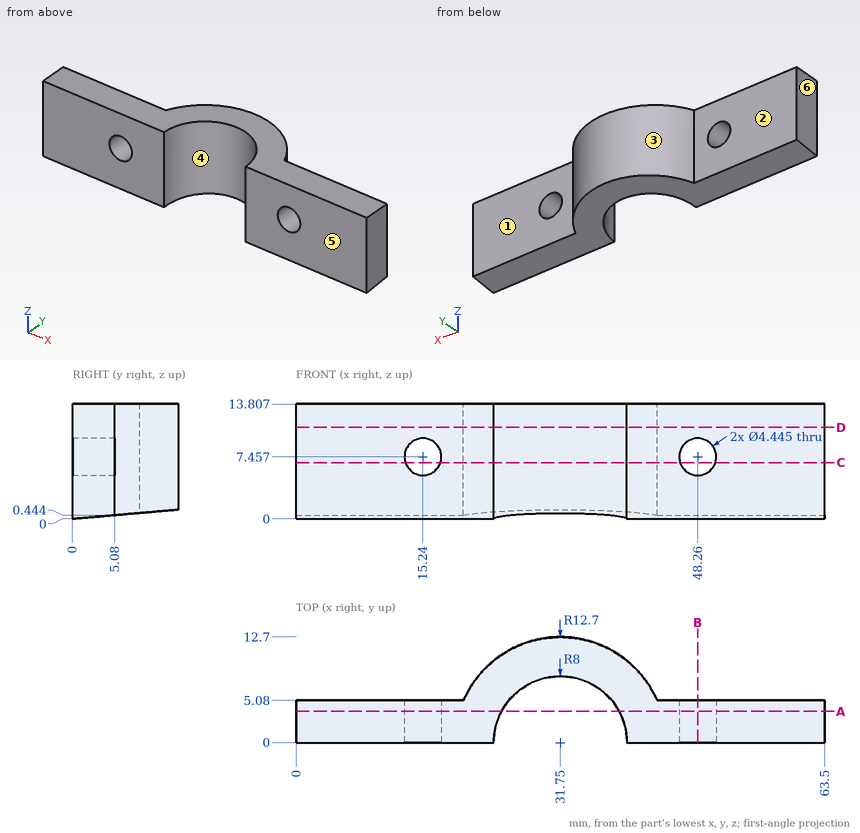
Input: dimensioned drawing with shaded views. Units: mm. Origin: part minimum x, y, z. A direction names the side the tool comes from. Coordinates: 2 decimals unless noted, no trailing zeros. Order: outer loops, then holes, each group sorted by start corner. A loop starts at its lowest first (then second) coordinate and runs counter-clockwise, first axis right, second up. Notation, with made-up numbers: M -31,49 L -2,49 A21 ccw -2,57 Z; hole C -4,82 d8. An arc over 180 degrees is marked long. Answer as CSV lines item,"result".
Q1. Section B-B on x = 48.26. Return the cut outline in (y, z) (1 decimal).
Answers:
outline,"M 0,0 L 5.1,0.4 L 5.1,5.2 L 0,5.2 Z; M 0,9.7 L 5.1,9.7 L 5.1,13.8 L 0,13.8 Z"
Q2. Draft query along X for the marked faces 4, 5 and 6. Return one class per face: pulls with the +X half, pulls with the -X half, needs draft (parallel to the pull), parting line crosses it, or undercut.
Answers:
face 4,"undercut"
face 5,"needs draft"
face 6,"pulls with the -X half"
Q3. Line query: probe 1 along X at (y, z) = (4.25, 9); probe 2 along X at (y, z) = (4.25, 5.5) (1 decimal); probe 3 along Y at (x, z) = (44, 4.25). Output: solid intervals per line, ascending. Write a range as [from, to].
Answers:
probe 1,"x = [0, 13.64], [16.84, 24.97], [38.53, 46.66], [49.86, 63.5]"
probe 2,"x = [0, 14.2], [16.3, 25], [38.5, 47.2], [49.3, 63.5]"
probe 3,"y = [0, 5.08]"
Q4. Section A-A on y = 3.75. Return the cut outline in (x, z) (1 decimal).
Answers:
outline,"M 0,0.3 L 24.7,0.3 L 24.7,13.8 L 0,13.8 Z; M 38.8,0.3 L 63.5,0.3 L 63.5,13.8 L 38.8,13.8 Z; hole C 15.2,7.5 d4.4; hole C 48.3,7.5 d4.4"
Q5. Section C-C on z = 6.75. Return the cut outline in (x, y).
Answers:
outline,"M 0,0 L 13.13,0 L 13.13,5.08 L 0,5.08 Z; M 17.35,0 L 23.75,0 A8 cw 39.75,0 L 46.15,0 L 46.15,5.08 L 43.39,5.08 A12.7 ccw 20.11,5.08 L 17.35,5.08 Z; M 50.37,0 L 63.5,0 L 63.5,5.08 L 50.37,5.08 Z"
Q6. Set-up query: the marked faces 1, 2 and 3. Return all of +Z, -Z, +X, -X, +Y, -Y with unobstructed straight access to the full face (end or side cutting, diameter ignored); none if empty.
Answers:
face 1,"+Z, -Z, +X, +Y"
face 2,"+Z, -Z, -X, +Y"
face 3,"+Z, -Z, +Y"
Q7. Section D-D on z = 11. Return the cut outline in (x, y), and give its area (3 significant figures).
Answers:
outline,"M 0,0 L 23.75,0 A8 cw 39.75,0 L 63.5,0 L 63.5,5.08 L 43.39,5.08 A12.7 ccw 20.11,5.08 L 0,5.08 Z"
area,"350 mm^2"
Q8. First-contact query: P1, Ø4, axis at y = 8.5, z = 9.5, coming from the -X side; P2, Ø6, axis at x = 35, y = 8, coming from the -Z side; P3, Ø3, axis at y = 11, z = 12, coming from the -X side. Flat tips, straight axial feed; report the tip coordinate or a pass-through.
Answers:
P1,"stops at x = 20.84"
P2,"stops at z = 0.52"
P3,"stops at x = 23.32"
